Verification items for the finished model (mm, model axes). A direction names the side the tool comes from. Coordinates: 2 decimals unless noted, no trailing zeros. Order: outer loops, then holes, each group sorted by start corner. A loop starts at its lowest first (then second) coordinate and runs counter-clockwise, first axis right, second up. Notation, with made-up numbers: (-27.5, 15) -> (24.5, 15) arc R16 cw to (24.5, 21) -> close; hole circle Ø2 at (62.25, 79.25). An arc over 180 degrees is marked (long way). Use CSV: the item, a comma, the result in double quotes. Start each with the question number.
1) Release check for a two-part mould opening along Z. For faces 1 (the cylindrical face through (31.732, 1.144, -71.228)), 2 (the cylindrical face through (-15.895, 18.241, -61.452)), 3 (the flat face through (18, -1, -74.447)), 4 (the flat face through (27, 9, -68.097)) record: released by +Z, released by -Z, zero draft, split by the parting line, or undercut.
2) Tool access check on faces 5 (the cylindrical face through (-14.3, -13.35, -42.34)), 6 (the cylindrical face through (4.66, 45.07, -23.09)), 7 (the flat face through (73.5, -15.3, -59.842)). Record the directions out of +Z, -Z, +X, -X, +Y, -Y that give a thin tool (end or side, any length) a straight path to the whole face; none if there is none.
3) Scan lines: line 1 along Y through (x, z) = (27, -61); line 2 along Z through (x, y) = (70, -25); line 3 along Y through (x, z) = (27, -45.5). Record each from-to range of solid material in increasing order.
4) Go/stop test with flat-tipped pins: pin 1 (4 mm diameter, centred on y = -31.5, z = -41.5, fed in from -X); pin 2 (12 mm diameter, centred on x = 35.5, z = -56, fed in from +Y); pin 3 (1.5 mm diameter, centred on x = 44, z = -63, fed in from -Y); pin 4 (4.5 mm diameter, centred on x = 28.1, y = 0, fed in from +Z). Record where each tip stops, or that it passes through.
5) Sectioned sample at C-C on z = -45.5. Record the boundary of the cut face in (x, y), then the cut area to 3 significant figures.
6) Sectioned sample at A-A on y = 0. Record the boundary of the cut face in (x, z), then the cut area to 3 significant figures.
7) Sectioned sample at B-B on x = -3. Record the boundary of the cut face in (y, z).
8) Sectioned sample at D-D on y = -43. Record the boundary of the cut face in (x, z).
from build123d import *

# Parameters (mm, degrees)
SKETCH3_R          = 3.81
CUT_EXTRUDE1_DEPTH = 107.706198127


with BuildPart() as part:
    # Sketch2 → Revolve1 (revolve)
    with BuildSketch(Plane(origin=(0, 0, 0), x_dir=(1, 0, 0), z_dir=(0, 1, 0))):
        Polygon((-16.351757188, 17.29715655), (-22.701757188, 17.29715655), (-22.701757188, 28.72715655), (-19.526757188, 28.72715655), (-19.526757188, 31.97835655), (-22.701757188, 31.97835655), (-22.701757188, 59.84215655), (-19.526757188, 59.84215655), (-19.526757188, 63.01715655), (-22.701757188, 63.01715655), (-22.701757188, 74.44715655), (28.098242812, 74.44715655), (28.098242812, 68.09715655), (-16.351757188, 68.09715655), align=None)
    revolve(axis=Axis((28.098242812, 0, -74.44715655), (0, 0, 1)))

    # Sketch3 → Cut-Extrude1 (cut, through all)
    with BuildSketch(Plane.XY.offset(-68.09715655)):
        with Locations((28.098242812, 0)):
            Circle(SKETCH3_R)
    extrude(amount=-CUT_EXTRUDE1_DEPTH, mode=Mode.SUBTRACT)


solid = part.part
Answers follow:
1,face 1,"zero draft"
1,face 2,"undercut"
1,face 3,"released by -Z"
1,face 4,"released by +Z"
2,face 5,"+Z"
2,face 6,"+Z, -Z"
2,face 7,"none"
3,line 1,"y = -47.61 to -44.44, 44.44 to 47.61"
3,line 2,"z = -74.45 to -63.02, -59.84 to -31.98, -28.73 to -17.3"
3,line 3,"y = -50.79 to -44.44, 44.44 to 50.79"
4,pin 1,"stops at x = -13.26"
4,pin 2,"stops at y = 50.78"
4,pin 3,"stops at y = -48.49"
4,pin 4,"passes through"
5,outline,"circle Ø101.6 at (28.1, 0); hole circle Ø88.9 at (28.1, 0)"
5,area,"1,900 mm²"
6,outline,"(-22.7, -74.45) -> (24.29, -74.45) -> (24.29, -68.1) -> (-16.35, -68.1) -> (-16.35, -17.3) -> (-22.7, -17.3) -> (-22.7, -28.73) -> (-19.53, -28.73) -> (-19.53, -31.98) -> (-22.7, -31.98) -> (-22.7, -59.84) -> (-19.53, -59.84) -> (-19.53, -63.02) -> (-22.7, -63.02) -> close; (31.91, -74.45) -> (78.9, -74.45) -> (78.9, -63.02) -> (75.72, -63.02) -> (75.72, -59.84) -> (78.9, -59.84) -> (78.9, -31.98) -> (75.72, -31.98) -> (75.72, -28.73) -> (78.9, -28.73) -> (78.9, -17.3) -> (72.55, -17.3) -> (72.55, -68.1) -> (31.91, -68.1) -> close"
6,area,"1,200 mm²"
7,outline,"(-40.17, -74.45) -> (40.17, -74.45) -> (40.17, -63.02) -> (36.07, -63.02) -> (36.07, -59.84) -> (40.17, -59.84) -> (40.17, -31.98) -> (36.07, -31.98) -> (36.07, -28.73) -> (40.17, -28.73) -> (40.17, -17.3) -> (31.76, -17.3) -> (31.76, -68.1) -> (-31.76, -68.1) -> (-31.76, -17.3) -> (-40.17, -17.3) -> (-40.17, -28.73) -> (-36.07, -28.73) -> (-36.07, -31.98) -> (-40.17, -31.98) -> (-40.17, -59.84) -> (-36.07, -59.84) -> (-36.07, -63.02) -> (-40.17, -63.02) -> close"
8,outline,"(1.05, -74.45) -> (55.15, -74.45) -> (55.15, -63.02) -> (48.57, -63.02) -> (48.57, -59.84) -> (55.15, -59.84) -> (55.15, -31.98) -> (48.57, -31.98) -> (48.57, -28.73) -> (55.15, -28.73) -> (55.15, -17.3) -> (39.36, -17.3) -> (39.36, -68.1) -> (16.84, -68.1) -> (16.84, -17.3) -> (1.05, -17.3) -> (1.05, -28.73) -> (7.63, -28.73) -> (7.63, -31.98) -> (1.05, -31.98) -> (1.05, -59.84) -> (7.63, -59.84) -> (7.63, -63.02) -> (1.05, -63.02) -> close"
